Design review of the part shown in the three views and the two pictorial views. Dimensions are in mm from the part's minimum x, y and z. Give positions to 0.01 mm unless a question says otherwise; leave off trailing zeros. Loops run counter-clockwise (first coordinate to the right, second up) from the corner with the lowest first, then second, coordinate; pieces in that order, holes last. Notation, with made-up numbers: (-4.75, 42) - (38.25, 42) arc R15 ccw to (38.25, 60) - close; hole circle Ø3 at (-18, -9.75). An arc over 180 degrees is marked (long way). Put each result on its own line as item: value. Start each with the question number.
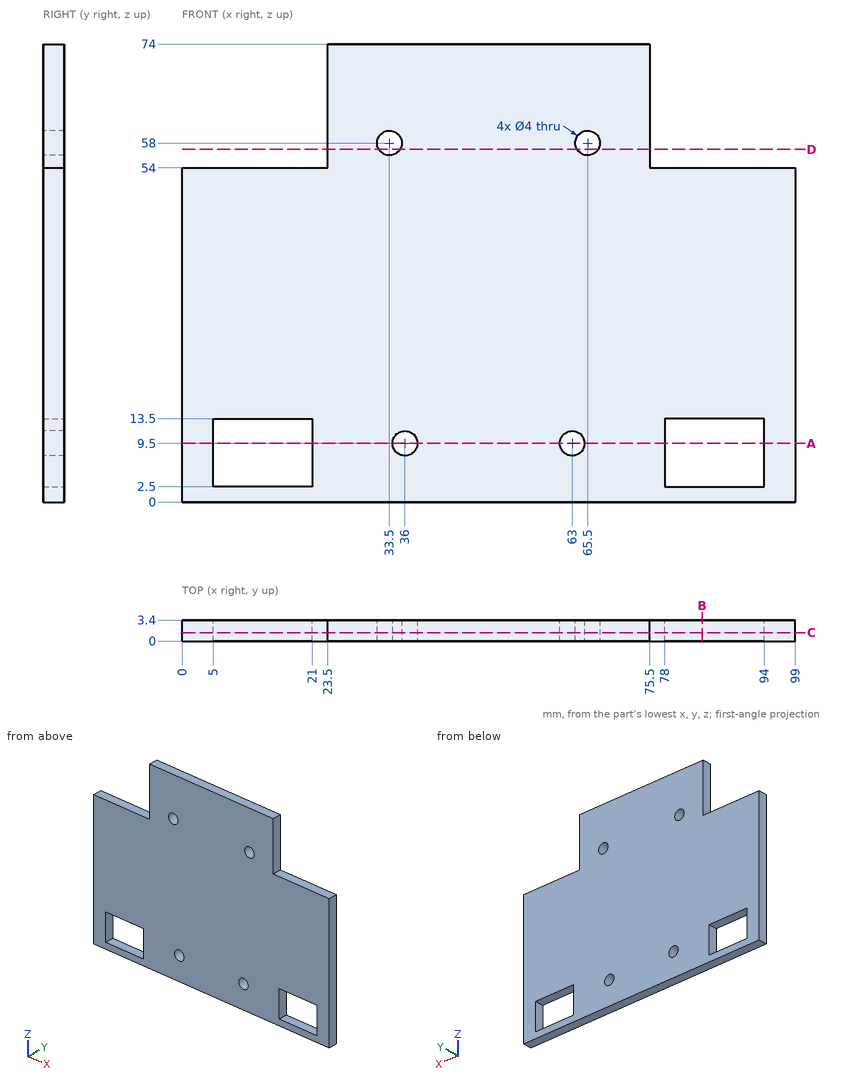
1) Wall thickness on probe 1 along X at (y, z) = (2.3, 5); probe 2 along Z at (x, y) = (65.5, 1.45); probe 3 along Z at (x, y) = (11.5, 2.75): over which ranges is each line inside the solid? List them lowest first.
2) Take a section at A-A on z = 9.5. State the section outline as (x, y) points, and give its area (3 significant figures).
3) Take a section at D-D on z = 57. State the section outline as (x, y) points, and give its area (3 significant figures).
4) Take a section at B-B on x = 84. State the section outline as (y, z) points, and give its area (3 significant figures).
5) Insertion check: P1, Ø1, axis at y = 2, z = 66, coming from the -X side; P2, Ø1, axis at x = 90.5, y = 1.5, coming from the +Z side. Each pin has a flat end and moves straight along its axis. Give the tip position at first contact, or say it passes through.
6) Take a section at C-C on y = 1.4. State the section outline as (x, z) points, and give its area (3 significant figures).
Answers follow:
1. probe 1: 0 to 5, 21 to 78, 94 to 99
1. probe 2: 0 to 56, 60 to 74
1. probe 3: 0 to 2.5, 13.5 to 54
2. outline: (0, 0) - (5, 0) - (5, 3.4) - (0, 3.4) - close; (21, 0) - (34, 0) - (34, 3.4) - (21, 3.4) - close; (38, 0) - (61, 0) - (61, 3.4) - (38, 3.4) - close; (65, 0) - (78, 0) - (78, 3.4) - (65, 3.4) - close; (94, 0) - (99, 0) - (99, 3.4) - (94, 3.4) - close
2. area: 201 mm2
3. outline: (23.5, 0) - (31.77, 0) - (31.77, 3.4) - (23.5, 3.4) - close; (35.23, 0) - (63.77, 0) - (63.77, 3.4) - (35.23, 3.4) - close; (67.23, 0) - (75.5, 0) - (75.5, 3.4) - (67.23, 3.4) - close
3. area: 153 mm2
4. outline: (0, 0) - (3.4, 0) - (3.4, 2.5) - (0, 2.5) - close; (0, 13.5) - (3.4, 13.5) - (3.4, 54) - (0, 54) - close
4. area: 146 mm2
5. P1: x = 23.5
5. P2: z = 54
6. outline: (0, 0) - (99, 0) - (99, 54) - (75.5, 54) - (75.5, 74) - (23.5, 74) - (23.5, 54) - (0, 54) - close; hole (5, 2.5) - (21, 2.5) - (21, 13.5) - (5, 13.5) - close; hole circle Ø4 at (33.5, 58); hole circle Ø4 at (36, 9.5); hole circle Ø4 at (63, 9.5); hole circle Ø4 at (65.5, 58); hole (78, 2.5) - (94, 2.5) - (94, 13.5) - (78, 13.5) - close
6. area: 5,980 mm2
